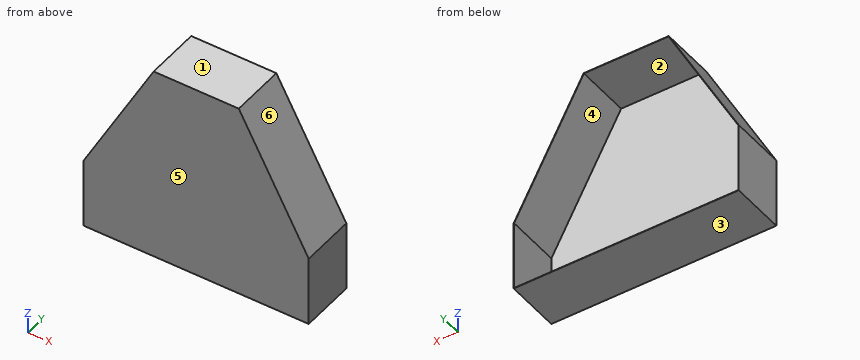
```python
from build123d import *

# Parameters (mm, degrees)
BOSS_EXTRUDE1_DEPTH = 135
SHELL1_T            = -2


with BuildPart() as part:
    # Sketch1 → Boss-Extrude1 (new, symmetric)
    with BuildSketch(Plane(origin=(0, 0, 0), x_dir=(1, 0, 0), z_dir=(0, 1, 0))):
        Polygon((550, 0), (-550, 0), (-550, -344), (-208, -974.384977503), (208, -974.384977503), (550, -344), align=None)
    extrude(amount=BOSS_EXTRUDE1_DEPTH, both=True)

    # Shell1
    shell1_openings = [part.faces().sort_by_distance(p)[0] for p in [
        (0, 135, 417.430162071),
    ]]
    offset(amount=SHELL1_T, openings=shell1_openings, kind=Kind.INTERSECTION)


solid = part.part
```
Input: part model. Units: mm. Frame: model coordinates. Face numbers are marked on the shaded views. A direction names the side the tool comes from. Round coordinates to 2 decimals unless told otherwise and drop trailing zeros. Loops run counter-clockwise (first coordinate to the right, second up) from the corner with the lowest first, then second, coordinate; pieces in that order, holes last. Notation, with made-up numbers: M 32,-1 L 64,-1 A21 ccw 64,21 Z; hole C 23,54.25 d5. An arc over 180 degrees is marked long. Answer in a Markdown table with one row per item. Add a question column.
1. Mould query, pull axis Z, two halves, no side actions, for the marked faces 3, 4, 5 and 6. Classes: released by +Z, released by -Z, zero draft, split by the parting line, or undercut.
2. Section C-C (x = -3.5). Output: boundary loops of the cut face in (y, z), and give its area (3 significant figures).
3. Section B-B (y = -112). Output: boundary loops of the cut face in (x, z), and give its area (3 significant figures).
4. Section A-A (z = 82). Output: boundary loops of the cut face in (x, y).
5. Contact query for flat-ended pins moving along their axis: pin 1 (4 mm diameter, centred on y = 31, z = 547.5, fed in from -X); pin 2 (1.5 mm diameter, centred on x = -429.5, y = 51.5, fed in from +Z); pin 3 (10 mm diameter, centred on y = 80, z = 492, fed in from +X). Output: stop coordinate, or through.
6. Ray query, probe 1 along Z at (x, y) = (-183, 120.5); probe 2 along X at (y, z) = (-38, 322); probe 3 along Y at (x, z) = (287, 816.5). Return the intervals inside material, ascending.
7. Set-up query: the marked faces 1 and 2. Return all of +Z, -Z, +X, -X, +Y, -Y with unobstructed straight access to the full face (end or side cutting, diameter ignored); none if empty.
Values follow:
| question | item | result |
|---|---|---|
| 1 | face 3 | released by -Z |
| 1 | face 4 | undercut |
| 1 | face 5 | zero draft |
| 1 | face 6 | released by +Z |
| 2 | outline | M -135,0 L 135,0 L 135,2 L -133,2 L -133,972.38 L 135,972.38 L 135,974.38 L -135,974.38 Z |
| 2 | area | 3,020 mm^2 |
| 3 | outline | M -550,0 L 550,0 L 550,344 L 208,974.38 L -208,974.38 L -550,344 Z; hole M -548,2 L 548,2 L 548,343.49 L 206.81,972.38 L -206.81,972.38 L -548,343.49 Z |
| 3 | area | 7,260 mm^2 |
| 4 | outline | M -550,-135 L 550,-135 L 550,135 L 548,135 L 548,-133 L -548,-133 L -548,135 L -550,135 Z |
| 5 | pin 1 | x = -440.68 |
| 5 | pin 2 | z = 567.49 |
| 5 | pin 3 | x = 472.42 |
| 6 | probe 1 | 0 to 2, 972.38 to 974.38 |
| 6 | probe 2 | -550 to -548, 548 to 550 |
| 6 | probe 3 | -135 to -133 |
| 7 | face 1 | +Z, +X, -X, +Y, -Y |
| 7 | face 2 | +Y |
